The listing builds one solid part. Answer for the finished solid, in the listing's coordinates (mm). Round coordinates to 2 decimals unless told otherwise and drop trailing zeros. Order: outer loops, then holes, each group sorted by start corner. A loop starts at its lowest first (then second) coordinate and runs counter-clockwise, first axis right, second up. Notation, with made-up numbers: (85, -2) -> (134, -2) arc R22 ccw to (134, 14) -> close; hole circle Ø2 at (-18, -39). An arc over 180 degrees is marked (long way). Return JSON: item names as keys, results as strings. Group by question number.
(1) Consider line 1 (Y direction, x = 73.5, z = 3.8); line 2 (Y direction, x = -16.5, z = 1.2). Determine where each line is inside the solid, lowest interval first. Write a range as [from, to].
(2) Determine the mould class of faces 1 (the face through (-62.251, 4.615, 2.465)), 2 (the face through (1, 14, 2)), 3 (the face through (94.5, 7, 2)), 4 (the face through (71.517, 7.26, 2.465)) for opening direction Y: +Y half, -Y half, draft (parallel to the pull), parting line (faces both ways), or undercut.
(3) The part is cut by section C-C (x = -16.5). Determine the outline of the cut face in (y, z).
(4) The part is cut by section B-B (z = 1.9). Determine the outline of the cut face in (x, y).
(5) This flat-tipped pin is pushed along its axis until it touches: pin 1 (5 mm diameter, centred on x = -26, y = 8, fed in from -Z). Where does it stop, or does it pass through?
(6) The part is cut by section A-A (x = 35.5). Determine the outline of the cut face in (y, z), plus the area to 3 significant figures.
Autodesk Inventor part; units mm, degrees
ref_plane "YZ Plane" through (0, 0, 0) normal (1, 0, 0) x (0, 1, 0)
ref_plane "XZ Plane" through (0, 0, 0) normal (0, 1, 0) x (-1, 0, 0)
ref_plane "XY Plane" through (0, 0, 0) normal (0, 0, 1) x (1, 0, 0)
sketch "Sketch1" plane through (0, 0, 0) normal (0, 0, 1) x (1, 0, 0)
  line L0 (-94.5, 0) -> (94.5, 0)
  line L1 (94.5, 0) -> (94.5, 14)
  line L2 (94.5, 14) -> (-94.5, 14)
  line L3 (-94.5, 14) -> (-94.5, 0)
  point P0 (0, 0)
  point P1 (0, 0)
  dimension "d0" = 14
  dimension "d1" = 189
extrude "Extrusion1" add sketch "Sketch1" along normal blind 5
sketch "Sketch2" plane through (0, 0, 5) normal (0, 0, 1) x (1, 0, 0)
  line L0 (94.5, 0) -> (94.5, 14)
  line L1 (-94.5, 0) -> (94.5, 0)
  point P0 (0, 0)
  point P1 (-61.5, 7)
  point P2 (-16.5, 7)
  point P3 (88.5, 7)
  dimension "d4" = 6
  dimension "d5" = 7
  dimension "d6" = 105
  dimension "d7" = 45
hole "Hole1" at (-61.5, 7, 5) at (-16.5, 7, 5) at (88.5, 7, 5) direction (0, 0, -1) diameter 5 depth 5
sketch "Sketch3" plane through (0, 0, 5) normal (0, 0, 1) x (1, 0, 0)
  line L0 (-94.5, 0) -> (94.5, 0)
  circle A0 centre (88.5, 7) radius 2.5
  circle A1 centre (-61.5, 7) radius 2.5
  point P0 (0, 0)
  point P1 (73.5, 7)
  point P2 (35.5, 7)
  point P3 (-76.5, 7)
  point P4 (-90.5, 7)
  dimension "d22" = 7
  dimension "d23" = 15
  dimension "d24" = 38
  dimension "d25" = 15
  dimension "d26" = 14
hole "Hole2" at (73.5, 7, 5) at (35.5, 7, 5) at (-76.5, 7, 5) at (-90.5, 7, 5) direction (0, 0, -1) diameter 4 depth 5
properties part number "144" material "Stainless Steel"
Answer below:
{
 "1": {"line 1": "y = [0, 5], [9, 14]", "line 2": "y = [0, 4.5], [9.5, 14]"},
 "2": {"face 1": "undercut", "face 2": "+Y half", "face 3": "draft", "face 4": "undercut"},
 "3": {"outline": "(0, 0) -> (4.5, 0) -> (4.5, 5) -> (0, 5) -> close; (9.5, 0) -> (14, 0) -> (14, 5) -> (9.5, 5) -> close"},
 "4": {"outline": "(-94.5, 0) -> (94.5, 0) -> (94.5, 14) -> (-94.5, 14) -> close; hole circle Ø4 at (-90.5, 7); hole circle Ø4 at (-76.5, 7); hole circle Ø5 at (-61.5, 7); hole circle Ø5 at (-16.5, 7); hole circle Ø4 at (35.5, 7); hole circle Ø4 at (73.5, 7); hole circle Ø5 at (88.5, 7)"},
 "5": {"pin 1": "stops at z = 0"},
 "6": {"outline": "(0, 0) -> (5, 0) -> (5, 5) -> (0, 5) -> close; (9, 0) -> (14, 0) -> (14, 5) -> (9, 5) -> close", "area": "50.0 mm²"}
}
